```python
from build123d import *

# Parameters (mm, degrees)
BOSS_EXTRUDE1_DEPTH   = 1.6
SKETCH2_R             = 3.45
BOSS_EXTRUDE2_DEPTH   = 1.4
M5X0_8_TAPPED_HOLE1_D = 4.2
BOSS_EXTRUDE3_DEPTH   = 5


with BuildPart() as part:
    # Sketch1 → Boss-Extrude1 (new body)
    with BuildSketch(Plane.XY):
        with BuildLine():
            Line((-3.5, 2), (-2.5, 2))
            Line((-2.5, 2), (-2.5, 0))
            Line((-2.5, 0), (2.5, 0))
            Line((2.5, 0), (2.5, 2))
            Line((2.5, 2), (3.5, 2))
            ThreePointArc((3.5, 2), (4.560660172, 2.439339828), (5, 3.5))
            Line((5, 3.5), (5, 29.5))
            Line((5, 29.5), (3.841886117, 32.974341649))
            ThreePointArc((3.841886117, 32.974341649), (3.295926597, 33.716863278), (2.41886117, 34))
            Line((2.41886117, 34), (-2.41886117, 34))
            ThreePointArc((-2.41886117, 34), (-3.295926597, 33.716863278), (-3.841886117, 32.974341649))
            Line((-3.841886117, 32.974341649), (-5, 29.5))
            Line((-5, 29.5), (-5, 3.5))
            ThreePointArc((-5, 3.5), (-4.560660172, 2.439339828), (-3.5, 2))
        make_face()
    boss_extrude1 = extrude(amount=BOSS_EXTRUDE1_DEPTH)

    # Sketch2 → Boss-Extrude2 (add)
    with BuildSketch(Plane.XY.offset(1.6)):
        with Locations((0, 6.96)):
            Circle(SKETCH2_R)
        with Locations((0, 26.96)):
            Circle(SKETCH2_R)
    boss_extrude2 = extrude(amount=BOSS_EXTRUDE2_DEPTH)

    # M5x0.8 Tapped Hole1 (through all)
    with Locations(Plane.XY.offset(3)):
        with Locations((0, 26.96), (0, 6.96)):
            m5x0_8_tapped_hole1 = Hole(M5X0_8_TAPPED_HOLE1_D / 2)

    # Sketch5 → Boss-Extrude3 (add)
    with BuildSketch(Plane(origin=(2.5, 0, 0), x_dir=(0, 0, -1), z_dir=(1, 0, 0))):
        with BuildLine():
            Line((0, 0), (-1.6, 0))
            ThreePointArc((-1.6, 0), (-1.13137085, -1.13137085), (0, -1.6))
            Line((0, -1.6), (0, 0))
        make_face()
    extrude(amount=-BOSS_EXTRUDE3_DEPTH)

    # Mirror4: Boss-Extrude1, Boss-Extrude2, M5x0.8 Tapped Hole1 across plane
    add(boss_extrude1.mirror(Plane(origin=(0, 0, 0), x_dir=(0, -0.707106781, 0.707106781), z_dir=(0, -0.707106781, -0.707106781))))
    add(boss_extrude2.mirror(Plane(origin=(0, 0, 0), x_dir=(0, -0.707106781, 0.707106781), z_dir=(0, -0.707106781, -0.707106781))))
    add(m5x0_8_tapped_hole1.mirror(Plane(origin=(0, 0, 0), x_dir=(0, -0.707106781, 0.707106781), z_dir=(0, -0.707106781, -0.707106781))), mode=Mode.SUBTRACT)


solid = part.part
```
Can you work these out from the model? Positions are in its coordinate system, mm. A direction names the side the tool comes from. Round coordinates to 2 decimals unless told otherwise and drop trailing zeros. Loops run counter-clockwise (first coordinate to the right, second up) from the corner with the lowest first, then second, coordinate; pieces in that order, holes last. Notation, with made-up numbers: (48.25, -22.75) -> (84.25, -22.75) arc R33 cw to (84.25, 5.25) -> close; hole circle Ø11 at (-1.75, -22.75). An arc over 180 degrees is marked (long way). Answer in a Markdown table with one row per item.
Item 1: If I drill on probe 1 along Y at (x, z) = (0, 2); probe 2 along Z at (x, y) = (0, -2.25); probe 3 along X at (y, z) = (-1.7, -26.96), over which ranges is the centre line in solid material (lowest first)?
Answer block:
| item | result |
|---|---|
| probe 1 | 3.51 to 4.86, 9.06 to 10.41, 23.51 to 24.86, 29.06 to 30.41 |
| probe 2 | -30.41 to -29.06, -24.86 to -23.51, -10.41 to -9.06, -4.86 to -3.51 |
| probe 3 | -3.45 to -2.1, 2.1 to 3.45 |
Item 2: Will these pins go through, and if not, where does the flat tip stop? P1, Ø0.5, axis at x = -3, z = 0.5, coming from the -Y side; P2, Ø3, axis at y = 0.5, z = -0.5, coming from the -X side; P3, Ø0.5, axis at x = 3, y = -1, coming from the +Z side.
Answer block:
| item | result |
|---|---|
| P1 | y = 2 |
| P2 | x = -2.5 |
| P3 | z = -2 |
Item 3: Suppose I cut it at B-B, the plane y = 26.96. List the corners of the cut face in (x, z) for me, plus the area to 3 significant figures.
Answer block:
| item | result |
|---|---|
| outline | (-5, 0) -> (-2.1, 0) -> (-2.1, 3) -> (-3.45, 3) -> (-3.45, 1.6) -> (-5, 1.6) -> close; (2.1, 0) -> (5, 0) -> (5, 1.6) -> (3.45, 1.6) -> (3.45, 3) -> (2.1, 3) -> close |
| area | 13.1 mm² |
Item 4: Suppose I cut it at A-A, the plane z = -6.96. List the corners of the cut face in (x, y) for me, plus the area to 3 significant figures.
Answer block:
| item | result |
|---|---|
| outline | (-5, -1.6) -> (-3.45, -1.6) -> (-3.45, -3) -> (-2.1, -3) -> (-2.1, 0) -> (-5, 0) -> close; (2.1, -3) -> (3.45, -3) -> (3.45, -1.6) -> (5, -1.6) -> (5, 0) -> (2.1, 0) -> close |
| area | 13.1 mm² |
Item 5: On a 3-axis mill with a long thin cutter (end or side, diameter ignored), from which of +Z, -Z, +X, -X, +Y, -Y can I reach the whole of each face in a straight line? I mean faces 4 (the cylindrical face through (-0.748, -2.29, -3.592)), 5 (the flat face through (0, 17, 0)), 6 (the flat face through (0, 17, 1.6)), 7 (the flat face through (-2.5, -0.2, 0.2)). Say none if no direction works.
Answer block:
| item | result |
|---|---|
| face 4 | -Y |
| face 5 | -Z, +X, -X, +Y |
| face 6 | +Z |
| face 7 | +Z, -X, -Y |
Item 6: We'd pull the mould along Y, two halves only. Please class faces 1 (the flat face through (-4.4, 31.3, 0.8)), 2 (the cylindrical face through (-0.748, 23.592, 2.29)), 3 (the flat face through (-3, -1, -2)): released by +Y, released by -Y, zero draft, split by the parting line, or undercut.
Answer block:
| item | result |
|---|---|
| face 1 | released by +Y |
| face 2 | undercut |
| face 3 | zero draft |
Item 7: Suppose I cut it at C-C, the plane x = 0. Give the number of separate pieces and of enclosed holes in the cut face, plus the area to 3 significant figures.
Answer block:
| item | result |
|---|---|
| separate pieces | 5 |
| enclosed holes | 0 |
| area | 99.1 mm² |
Item 8: Suppose I cut it at D-D, the plane y = 15.5. List the corners of the cut face in (x, z) for me.
Answer block:
| item | result |
|---|---|
| outline | (-5, 0) -> (5, 0) -> (5, 1.6) -> (-5, 1.6) -> close |
